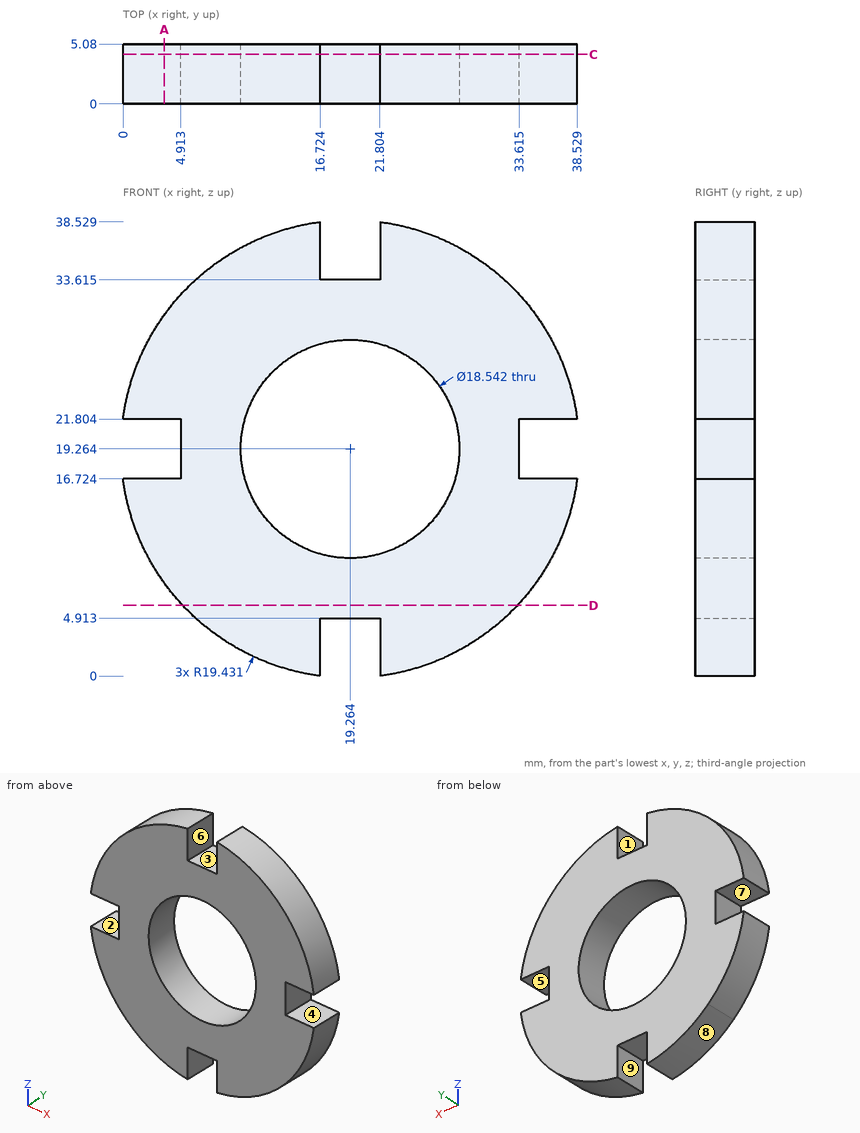
Design review of the part shown in the three views and the two pictorial views. Dimensions are in mm from the part's minimum x, y and z. A direction names the side the tool comes from. Round coordinates to 2 decimals unless told otherwise and drop trailing zeros. Order: outer loops, then holes, each group sorted by start corner. A loop starts at its lowest first (then second) coordinate and runs counter-clockwise, first axis right, second up. Notation, with made-up numbers: (-36, 10) -> (11, 10) arc R25 ccw to (11, 29) -> close; hole circle Ø10 at (-36, 30). An arc over 180 degrees is marked (long way). Write item = value, one per line. Start each with the question number.
1) Take a section at A-A on x = 3.5. State the section outline as (y, z) points (1 decimal).
2) Insertion check: pin 1 (1.5 mm diameter, centred on x = 3.5, y = 4, fed in from +Z); pin 2 (1 mm diameter, centred on x = 10, y = 2.5, fed in from -Z); pin 3 (1 mm diameter, centred on x = 23.5, y = 4, fed in from -Z) (1 decimal); pin 4 (5 mm diameter, centred on x = 34, z = 26.5, fed in from -Y). Each pin has a flat end and moves straight along its axis. Give the tip position at first contact, or say it passes through.
3) The part is to be moulded in two halves that separate along Z. For the marked faces 1, 2, 3 and 4, say which applies: +Z half, -Z half, draft (parallel to the pull), parting line (faces both ways), or undercut.
4) Tool access review of the marked faces 5, 6, 7, 8 and 9: name each direction out of +Z, -Z, +X, -X, +Y, -Y from which nothing blocks a thin tool from reaching the whole face with its end or side.
5) To check wall thickness, follow line 1 (Z direction, x = 18, y = 2.1) (1 decimal); line 2 (Z direction, x = 25.5, y = 4.35) (1 decimal); line 3 (X direction, y = 2.8, z = 27.5) (1 decimal). State the ranges of each line that lie inside material, in increasing order. Write a range as from..to.
6) Take a section at D-D on z = 6. State the section outline as (x, y) points (1 decimal).
7) Take a section at C-C on y = 4.2. State the section outline as (x, z) points (1 decimal).
Verdict:
q1.outline = (0, 7.9) -> (5.1, 7.9) -> (5.1, 16.7) -> (0, 16.7) -> close; (0, 21.8) -> (5.1, 21.8) -> (5.1, 30.6) -> (0, 30.6) -> close
q2.pin_1 = 31.6
q2.pin_2 = 1.92
q2.pin_3 = 0.2
q2.pin_4 = 0
q3.face_1 = draft
q3.face_2 = undercut
q3.face_3 = +Z half
q3.face_4 = undercut
q4.face_5 = +X, +Y, -Y
q4.face_6 = +Z, +Y, -Y
q4.face_7 = -X, +Y, -Y
q4.face_8 = -Z, -X, +Y, -Y
q4.face_9 = -Z, +Y, -Y
q5.line_1 = 4.9..10.1, 28.4..33.6
q5.line_2 = 0.9..12.4, 26.1..37.7
q5.line_3 = 1.7..15, 23.5..36.9
q6.outline = (5.1, 0) -> (33.5, 0) -> (33.5, 5.1) -> (5.1, 5.1) -> close
q7.outline = (0, 16.7) arc R19.4 ccw to (6.2, 4.9) arc R19.4 ccw to (16.7, 0) -> (16.7, 4.9) -> (21.8, 4.9) -> (21.8, 0) arc R19.4 ccw to (38.5, 16.7) -> (33.6, 16.7) -> (33.6, 21.8) -> (38.5, 21.8) arc R19.4 ccw to (21.8, 38.5) -> (21.8, 33.6) -> (16.7, 33.6) -> (16.7, 38.5) arc R19.4 ccw to (0, 21.8) -> (4.9, 21.8) -> (4.9, 16.7) -> close; hole circle Ø18.5 at (19.3, 19.3)
